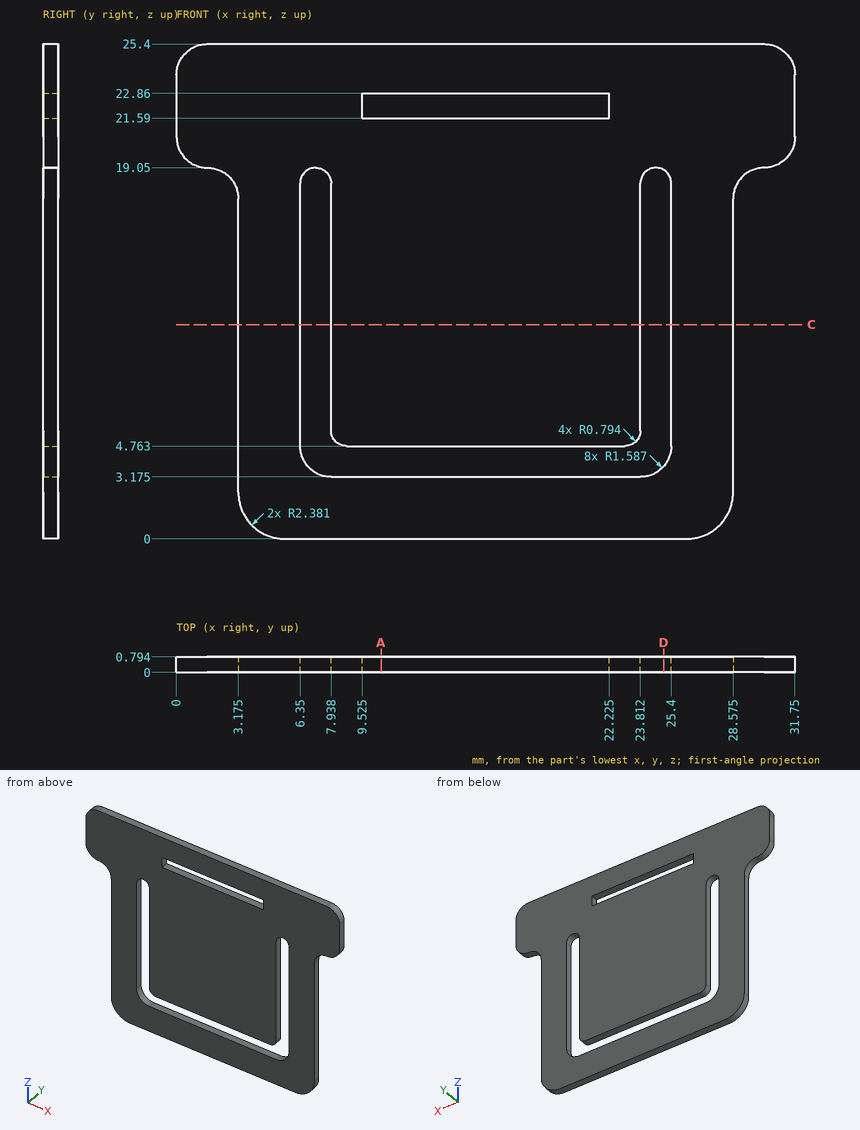
Geometry check sheet. Reference: drawing and pictorial views, mm from the part's lowest x, y, z. Coordinates: 2 decimals unless noted, no trailing zeros. Order: outer loops, then holes, each group sorted by start corner. A loop starts at its lowest first (then second) coordinate and runs counter-clockwise, first axis right, second up. Notation, with made-up numbers: M 77,-25.5 L 110,-25.5 A19 ccw 110,-3.5 Z; hole C 69.25,-38.75 d3. An arc over 180 degrees is marked long. Return JSON: item names as keys, results as strings.
1) Gauge pin test, flat end, axial feed: pin 1 (10 mm diameter, centred on x = 11, z = 6, fed in from -Y). Record the tip position at first contact, or that the pin passes through.
Answer list:
{"pin 1": "y = 0"}
2) Cross-section at C-C, the plane z = 11. Count the separate pieces of the cut face and the enclosed holes in it.
Answer list:
{"separate pieces": "3", "enclosed holes": "0"}
3) Cross-section at A-A, the plane x = 10.5. Record the boundary of the cut face in (y, z) (1 decimal).
Answer list:
{"outline": "M 0,0 L 0.8,0 L 0.8,3.2 L 0,3.2 Z; M 0,4.8 L 0.8,4.8 L 0.8,21.6 L 0,21.6 Z; M 0,22.9 L 0.8,22.9 L 0.8,25.4 L 0,25.4 Z"}
4) Cross-section at D-D, the plane x = 25. Record the boundary of the cut face in (y, z) (1 decimal).
Answer list:
{"outline": "M 0,0 L 0.8,0 L 0.8,3.7 L 0,3.7 Z; M 0,18.9 L 0.8,18.9 L 0.8,25.4 L 0,25.4 Z"}
5) Thickness scan on L1, parallel to Z at x = 10, y = 0.2 (1 decimal); L2, parallel to X at y = 0.7, z = 18; L3, parallel to X at y = 0.4, z = 18.5. Record the ranges inside material, lowest first. Write a range as [from, to].
Answer list:
{"L1": "[0, 3.2], [4.8, 21.6], [22.9, 25.4]", "L2": "[3.08, 6.35], [7.94, 23.81], [25.4, 28.67]", "L3": "[2.79, 6.39], [7.9, 23.85], [25.36, 28.96]"}
